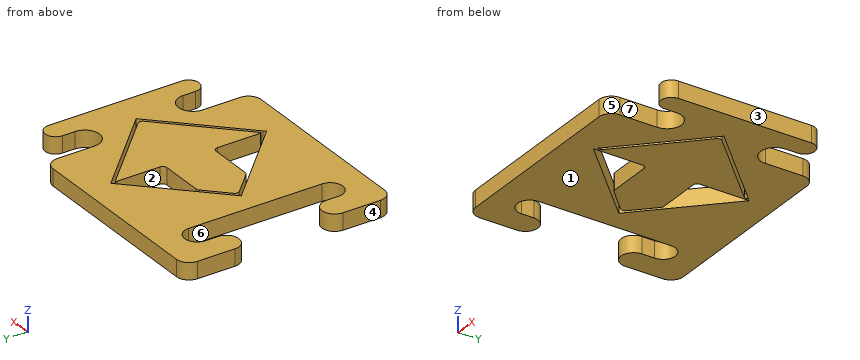
```python
from build123d import *

# Parameters (mm, degrees)
PAD_DEPTH       = 4
POCKET_DEPTH    = 4.001
POCKET001_DEPTH = 3
FILLET_R        = 0.2
FILLET001_R     = 0.2
FILLET002_R     = 1


with BuildPart() as part:
    # Sketch002 → Pad (new body)
    with BuildSketch(Plane.XY):
        with BuildLine():
            ThreePointArc((-5, -13), (-8.5, -9.5), (-12, -13))
            Line((-12, -22), (-12, -13))
            ThreePointArc((-15, -25), (-12.87868, -24.12132), (-12, -22))
            Line((-59, -25), (-15, -25))
            ThreePointArc((-62, -22), (-61.12132, -24.12132), (-59, -25))
            Line((-62, -13), (-62, -22))
            ThreePointArc((-56, -13), (-59, -10), (-62, -13))
            Line((-56, -13), (-56, -16))
            ThreePointArc((-56, -16), (-53, -19), (-50, -16))
            Line((-50, 16), (-50, -16))
            ThreePointArc((-50, 16), (-53, 19), (-56, 16))
            Line((-56, 13), (-56, 16))
            ThreePointArc((-62, 13), (-59, 10), (-56, 13))
            Line((-62, 22), (-62, 13))
            ThreePointArc((-59, 25), (-61.12132, 24.12132), (-62, 22))
            Line((-15, 25), (-59, 25))
            ThreePointArc((-12, 22), (-12.87868, 24.12132), (-15, 25))
            Line((-12, 22), (-12, 13))
            ThreePointArc((-12, 13), (-8.5, 9.5), (-5, 13))
            Line((-5, 13), (-5, 16))
            ThreePointArc((0, 16), (-2.5, 18.5), (-5, 16))
            Line((0, -16), (0, 16))
            ThreePointArc((-5, -16), (-2.5, -18.5), (0, -16))
            Line((-5, -13), (-5, -16))
        make_face()
    extrude(amount=PAD_DEPTH)

    # Sketch001 (on Face26 of Pad) → Pocket (cut, through all)
    with BuildSketch(Plane.XY.offset(4)):
        Polygon((-45, 0), (-26.260408, 18.739592), (-26.260408, 17.739592), (-26.260408, 5.913197), (-38.086803, 5.913197), (-44, 0), (-38.086803, -5.913197), (-26.260408, -5.913197), (-26.260408, -17.739592), (-26.260408, -18.739592), align=None)
        Polygon((-7.520815, 0), (-25.760408, 18.239592), (-25.760408, 17.239592), (-8.520815, 0), (-25.760408, -17.239592), (-25.760408, -18.239592), align=None)
    extrude(amount=-POCKET_DEPTH, mode=Mode.SUBTRACT)

    # Sketch (on Face5 of Pocket) → Pocket001 (cut)
    with BuildSketch(Plane.XY.offset(4)):
        Polygon((-25.760408, -17.239592), (-26.260408, -17.739592), (-26.260408, -18.739592), (-25.760408, -18.239592), align=None)
        Polygon((-26.260408, 18.739592), (-25.760408, 18.239592), (-25.760408, 17.239592), (-26.260408, 17.739592), align=None)
    extrude(amount=-POCKET001_DEPTH, mode=Mode.SUBTRACT)

    # Fillet
    fillet_edges = [part.edges().sort_by_distance(p)[0] for p in [
        (-26.260408, -17.739592, 2.5),
    ]]
    fillet(fillet_edges, radius=FILLET_R)

    # Fillet001
    fillet001_edges = [part.edges().sort_by_distance(p)[0] for p in [
        (-26.260408, 17.739592, 2.5),
    ]]
    fillet(fillet001_edges, radius=FILLET001_R)

    # Fillet002
    fillet002_edges = [part.edges().sort_by_distance(p)[0] for p in [
        (-44, 0, 2),
        (-38.086803, -5.913197, 2),
        (-38.086803, 5.913197, 2),
        (-26.260408, 5.913197, 2),
        (-26.260408, -5.913197, 2),
        (-8.520815, 0, 2),
    ]]
    fillet(fillet002_edges, radius=FILLET002_R)


solid = part.part
```
Work out the finished part from the listing and answer in its coordinate system (mm). Face numbers are marked on the shaded views. A direction names the side the tool comes from. Give positions to 0.01 mm unless a question says otherwise; leave off trailing zeros. Write each loop counter-clockwise with the first axis right and the second up, starting at its lowest first coordinate (ties: lowest second). Pieces come first, ordered by that corner, then holes. Notation, with made-up numbers: (1, 54) -> (51, 54) arc R28 ccw to (51, 86) -> close; hole circle Ø7 at (20, 46). An arc over 180 degrees is marked (long way). Write item = value, one per line.
Q1. Section C-C on z = 3.25 is taken. State how many separate pieces and enclosed holes the cut face has, and give its area (3 significant figures).
Computed values:
separate_pieces = 2
enclosed_holes = 1
area = 2,250 mm^2
Q2. Consider line 1 along Y through (x, z) = (-19, 2); line 2 along X through (y, z) = (-5, 2.75); line 3 along Y through (x, z) = (-53, 0.65). Determine where each line is inside the solid, lowest interval first.
Computed values:
line_1 = -25 to -11.48, -10.48 to 10.48, 11.48 to 25
line_2 = -50 to -40, -39 to -13.52, -12.52 to 0
line_3 = -25 to -19, 19 to 25
Q3. Section B-B on x = -30 is taken. Determine the outline of the cut face in (y, z), and give its area (3 significant figures).
Computed values:
outline = (-25, 0) -> (-15, 0) -> (-15, 4) -> (-25, 4) -> close; (-5.91, 0) -> (5.91, 0) -> (5.91, 4) -> (-5.91, 4) -> close; (15, 0) -> (25, 0) -> (25, 4) -> (15, 4) -> close
area = 127 mm^2
Q4. A tool of negligible diameter and unlimited length cuts with its end or side. For the marked faces 5, 6 and 7, from which of +Z, -Z, +X, -X, +Y, -Y can it reach the whole face along a straight path? Write none if from no direction.
Computed values:
face_5 = +Z, -Z, +X, -Y
face_6 = +Z, -Z
face_7 = +Z, -Z, -Y
Q5. Flat-ended cylindrical pins translate along their axes: pin 1 Ø0.5 at (y, z) = (18, 0.5) entering from +X; pin 2 Ø1.1 at (y, z) = (-18, 0.5) entering from +X. Find the tip coordinate at first contact, or state that the pin passes through.
Computed values:
pin_1 = -0.71
pin_2 = -0.46
Q6. Section D-D on y = 12 is taken. Determine the outline of the cut face in (x, z), and give its area (3 significant figures).
Computed values:
outline = (-61.83, 0) -> (-56.17, 0) -> (-56.17, 4) -> (-61.83, 4) -> close; (-50, 0) -> (-33, 0) -> (-33, 4) -> (-50, 4) -> close; (-26.26, 0) -> (-20.52, 0) -> (-20.52, 4) -> (-26.26, 4) -> close; (-19.52, 0) -> (-11.85, 0) -> (-11.85, 4) -> (-19.52, 4) -> close; (-5.15, 0) -> (0, 0) -> (0, 4) -> (-5.15, 4) -> close
area = 165 mm^2
Q7. For a pull along X with two mould halves and no side action, classify the marked faces 1, 2, 3 and 4 as pulls with the +X half, pulls with the -X half, needs draft (parallel to the pull), parting line crosses it, or undercut.
Computed values:
face_1 = needs draft
face_2 = undercut
face_3 = pulls with the +X half
face_4 = pulls with the -X half
Q8. Section A-A on x = -53 is taken. Determine the outline of the cut face in (y, z), and give its area (3 significant figures).
Computed values:
outline = (-25, 0) -> (-19, 0) -> (-19, 4) -> (-25, 4) -> close; (19, 0) -> (25, 0) -> (25, 4) -> (19, 4) -> close
area = 48.0 mm^2
